from build123d import *

# Parameters (mm, degrees)
BOSS_EXTRUDE1_DEPTH = 6.9
FILLET1_R           = 10
FILLET2_R           = 20
SKETCH3_R           = 2.5
CUT_EXTRUDE2_DEPTH  = 7.9
SKETCH2_R           = 3.85
CUT_EXTRUDE1_DEPTH  = 7.9


with BuildPart() as part:
    # Sketch1 → Boss-Extrude1 (new body)
    with BuildSketch(Plane(origin=(0, 0, 0), x_dir=(1, 0, 0), z_dir=(0, 1, 0))):
        Polygon((0, 0), (0, 100), (140, 100), (140, 60), (40, 60), (40, 0), align=None)
    extrude(amount=BOSS_EXTRUDE1_DEPTH)

    # Fillet1
    fillet1_edges = [part.edges().sort_by_distance(p)[0] for p in [
        (0, 3.45, 0),
        (140, 3.45, -100),
        (140, 3.45, -60),
        (40, 3.45, -60),
        (40, 3.45, 0),
    ]]
    fillet(fillet1_edges, radius=FILLET1_R)

    # Fillet2
    fillet2_edges = [part.edges().sort_by_distance(p)[0] for p in [
        (0, 3.45, -100),
    ]]
    fillet(fillet2_edges, radius=FILLET2_R)

    # Sketch3 → Cut-Extrude2 (cut, through all)
    with BuildSketch(Plane(origin=(0, 6.9, 0), x_dir=(1, 0, 0), z_dir=(0, 1, 0))):
        with Locations((20, 80)):
            Circle(SKETCH3_R)
    extrude(amount=-CUT_EXTRUDE2_DEPTH, mode=Mode.SUBTRACT)

    # Sketch2 → Cut-Extrude1 (cut, through all)
    with BuildSketch(Plane(origin=(0, 6.9, 0), x_dir=(1, 0, 0), z_dir=(0, 1, 0))):
        with Locations((20, 25)):
            Circle(SKETCH2_R)
        with Locations((115, 80)):
            Circle(SKETCH2_R)
    extrude(amount=-CUT_EXTRUDE1_DEPTH, mode=Mode.SUBTRACT)


solid = part.part
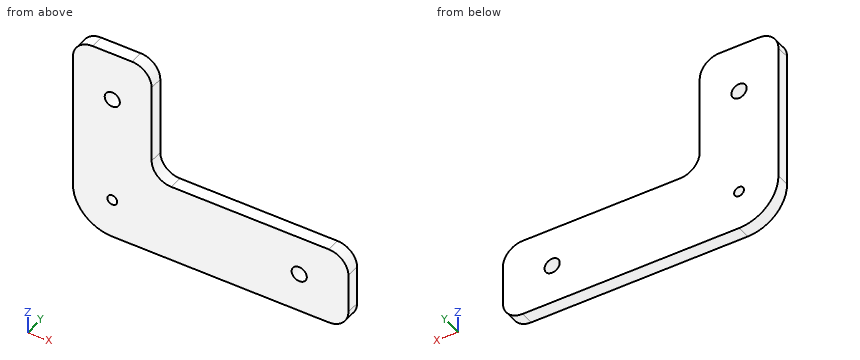
Geometry: final body of the model. Coordinates: model frame, mm. Give positions to 0.01 mm unless a question says otherwise; leave off trailing zeros. Order: outer loops, then holes, each group sorted by start corner. A loop starts at its lowest first (then second) coordinate and runs counter-clockwise, first axis right, second up. Notation, with made-up numbers: (-25, 68) -> (-2, 68) arc R21 ccw to (-2, 90) -> close; hole circle Ø4 at (55, 50.25). An arc over 180 degrees is marked (long way). Put each result on its own line as item: value.
Q1. Section B-B, the plane y = 5.75. Return loops of the section in (x, z).
Here are the results:
outline: (0, -80) arc R20 ccw to (20, -100) -> (130, -100) arc R10 ccw to (140, -90) -> (140, -70) arc R10 ccw to (130, -60) -> (50, -60) arc R10 cw to (40, -50) -> (40, -10) arc R10 ccw to (30, 0) -> (10, 0) arc R10 ccw to (0, -10) -> close; hole circle Ø7.7 at (20, -25); hole circle Ø5 at (20, -80); hole circle Ø7.7 at (115, -80)
Q2. Section C-C, the plane x = 115. Return loops of the section in (y, z).
Here are the results:
outline: (0, -100) -> (6.9, -100) -> (6.9, -83.85) -> (0, -83.85) -> close; (0, -76.15) -> (6.9, -76.15) -> (6.9, -60) -> (0, -60) -> close
Q3. Pin query (flat end, axial travel): pin 1 (3.5 mm diameter, centred on x = 102, y = 2, fed in from +Z); pin 2 (2 mm diameter, centred on x = 42, y = 4.5, fed in from +Z); pin 3 (8 mm diameter, centred on x = 42, z = -33.5, fed in from +Y); pin 4 (3.5 mm diameter, centred on y = 5, z = -23.5, fed in from +X). Return the tip coordinate at first contact, or that it passes through.
Here are the results:
pin 1: stops at z = -60
pin 2: stops at z = -54.36
pin 3: stops at y = 6.9
pin 4: stops at x = 40
Q4. Section A-A, the plane z = -25. Return loops of the section in (x, y), then the cut area to 3 significant figures.
Here are the results:
outline: (0, 0) -> (16.15, 0) -> (16.15, 6.9) -> (0, 6.9) -> close; (23.85, 0) -> (40, 0) -> (40, 6.9) -> (23.85, 6.9) -> close
area: 223 mm^2
Q5. Material intervals for L1, parallel to Z at x = 20, y = 2; L2, parallel to X at y = 4.25, z = -80; L3, parallel to Z at x = 115, y = 2, sorted ascending.
Here are the results:
L1: z = -100 to -82.5, -77.5 to -28.85, -21.15 to 0
L2: x = 0 to 17.5, 22.5 to 111.15, 118.85 to 140
L3: z = -100 to -83.85, -76.15 to -60
Q6. Section D-D, the plane x = 54.5. Return loops of the section in (y, z).
Here are the results:
outline: (0, -100) -> (6.9, -100) -> (6.9, -60) -> (0, -60) -> close
